from build123d import *
from OCP.BRepAlgoAPI import BRepAlgoAPI_Cut
from OCP.TopTools import TopTools_ListOfShape

# Parameters (mm, degrees)
BOSS_EXTRUDE1_START     = -164.670652
SKETCH1_R               = 7.9375
SKETCH1_R_2             = 6.4643
BOSS_EXTRUDE1_DEPTH     = 343.055109872
CUT_EXTRUDE1_DEPTH      = 179.737300592
CUT_EXTRUDE1_DEPTH_BACK = 179.737300592


with BuildPart() as part:
    # Sketch1 → Boss-Extrude1 (new body)
    with BuildSketch(Plane(origin=(0, 0, 0), x_dir=(1, 0, 0), z_dir=(0, 1, 0)).offset(BOSS_EXTRUDE1_START)):
        with Locations(Location((0, 0, 0), (0, 0, 270))):
            Circle(SKETCH1_R)
        with Locations(Location((0, 0, 0), (0, 0, 270))):
            Circle(SKETCH1_R_2, mode=Mode.SUBTRACT)
    extrude(amount=BOSS_EXTRUDE1_DEPTH)


with BuildPart() as cut_extrude1_tool:
    # Sketch2 → Cut-Extrude1 (new, two sides: drawn at the far end of the back side and taken through both)
    with BuildSketch(Plane.XY.offset(-CUT_EXTRUDE1_DEPTH_BACK)):
        with BuildLine():
            Line((-3.175, 178.384457539), (3.175, 178.384457539))
            Line((3.175, 178.384457539), (3.175, 152.984457539))
            ThreePointArc((3.175, 152.984457539), (2.710032015, 151.861925524), (1.5875, 151.396957539))
            Line((1.5875, 151.396957539), (-1.5875, 151.396957539))
            ThreePointArc((-1.5875, 151.396957539), (-2.710032015, 151.861925524), (-3.175, 152.984457539))
            Line((-3.175, 152.984457539), (-3.175, 178.384457539))
        make_face()
    extrude(amount=CUT_EXTRUDE1_DEPTH + CUT_EXTRUDE1_DEPTH_BACK)


with BuildPart() as part_1:
    add(part.part)

    # Cut-Extrude1: cut by cut_extrude1_tool, with a tolerance
    cut_extrude1_stock = TopTools_ListOfShape()
    cut_extrude1_stock.Append(part_1.part.wrapped)
    cut_extrude1_tools = TopTools_ListOfShape()
    cut_extrude1_tools.Append(cut_extrude1_tool.part.wrapped)
    cut_extrude1_cut = BRepAlgoAPI_Cut()
    cut_extrude1_cut.SetArguments(cut_extrude1_stock)
    cut_extrude1_cut.SetTools(cut_extrude1_tools)
    cut_extrude1_cut.SetFuzzyValue(0.00001)
    cut_extrude1_cut.Build()
    add(Compound.cast(cut_extrude1_cut.Shape()).solids(), mode=Mode.REPLACE)


solid = part_1.part
Could you check a few things on this model? Use its own coordinates, in mm. Round coordinates to 2 decimals unless told otherwise and drop trailing zeros. Write each loop counter-clockwise with the first axis right and the second up, starting at its lowest first coordinate (ties: lowest second). Pieces come first, ordered by that corner, then holes. Notation, with made-up numbers: (81.5, -5) - (92.5, -5) arc R21 cw to (92.5, 23) - close; hole circle Ø10 at (69.25, 51.5). An arc over 180 degrees is marked (long way). Use a Markdown table: item, result.
Q1. I want a section at B-B (y = 91). List the corners of the cut face in (x, z) for me (1 decimal), plus the area to 3 significant figures.
Output values:
| item | result |
|---|---|
| outline | circle Ø15.9 at (0, 0); hole circle Ø12.9 at (0, 0) |
| area | 66.7 mm2 |
Q2. I want a section at A-A (z = 0). List the corners of the cut face in (x, y) for me, plus the area to 3 significant figures.
Output values:
| item | result |
|---|---|
| outline | (-7.94, -164.67) - (-6.46, -164.67) - (-6.46, 178.38) - (-7.94, 178.38) - close; (6.46, -164.67) - (7.94, -164.67) - (7.94, 178.38) - (6.46, 178.38) - close |
| area | 1,010 mm2 |
Q3. Please list where these lines run through material, in increasing order: L1, parallel to X at y = 35.5, z = 0; L2, parallel to Z at x = 3.25, y = -38.5; L3, parallel to X at y = -115, z = -5.5.
Output values:
| item | result |
|---|---|
| L1 | -7.94 to -6.46, 6.46 to 7.94 |
| L2 | -7.24 to -5.59, 5.59 to 7.24 |
| L3 | -5.72 to -3.4, 3.4 to 5.72 |
Q4. For pin 1 (2 mm diameter, centred on y = -107, z = -3, fed in from +X); pin 2 (1.3 mm diameter, centred on y = 159.5, z = 6, fed in from +X); pin 3 (1.3 mm diameter, centred on y = 165.5, z = -6.5, fed in from +X); pin 4 (5 mm diameter, centred on x = -1, z = 4.5, fed in from +Y), each with a flat end and sliding along its axis, tell me the tip position at first contact or that it passes through.
Output values:
| item | result |
|---|---|
| pin 1 | x = 7.68 |
| pin 2 | x = 5.86 |
| pin 3 | x = 5.36 |
| pin 4 | y = 178.38 |
Q5. Thinking about a two-plate mould opening in X: for faces 1 (the cylindrical face through (0.35, 4.46, -7.93)), 2 (the flat face through (0, -164.671, -7)), 3 (the cylindrical face through (0.28, 4.46, -6.46)), which applies, released by +X, released by -X, zero draft, split by the parting line, or undercut?
Output values:
| item | result |
|---|---|
| face 1 | split by the parting line |
| face 2 | zero draft |
| face 3 | undercut |
